```python
from build123d import *

# Parameters (mm, degrees)
SKETCH_1_W              = 306
SKETCH_1_H              = 175
EXTRUDE_1_DEPTH         = 2
SKETCH_2_R              = 110
SKETCH_2_W              = 10
SKETCH_2_H              = 80
CUT_EXTRUDE_1_DEPTH     = 177.264715698
FILLET_1_R              = 5
HOLE_WIZARD_3_2_3_2_1_D = 3.2
HOLE_WIZARD_3_2_3_2_2_D = 3.2
CUT_EXTRUDE_2_DEPTH     = 10
FILLET_2_R              = 2
FILLET_2_OF_MIRROR_3_R  = 2


with BuildPart() as part:
    # 草图1 → 凸台-拉伸1 (new body)
    with BuildSketch(Plane.XY):
        Rectangle(SKETCH_1_W, SKETCH_1_H)
    extrude(amount=EXTRUDE_1_DEPTH)

    # 草图2 → 切除-拉伸1 (cut, through all)
    with BuildSketch(Plane.XY.offset(2)):
        with Locations((0, 87.5)):
            Circle(SKETCH_2_R)
        with Locations((-148, -7.5)):
            Rectangle(SKETCH_2_W, SKETCH_2_H)
        with Locations((148, -7.5)):
            Rectangle(SKETCH_2_W, SKETCH_2_H)
    extrude(amount=-CUT_EXTRUDE_1_DEPTH, mode=Mode.SUBTRACT)

    # 圆角1
    fillet_1_edges = [part.edges().sort_by_distance(p)[0] for p in [
        (143, -47.5, 1),
        (143, 32.5, 1),
        (-143, 32.5, 1),
        (-143, -47.5, 1),
    ]]
    fillet(fillet_1_edges, radius=FILLET_1_R)

    # Ø3.2 (3.2) 直径孔1 (through all)
    with Locations(Plane(origin=(-147, 82.5, 2), x_dir=(1, 0, 0), z_dir=(0, 0, 1))):
        with Locations((0, 0), (0, -20)):
            hole_wizard_3_2_3_2_1 = Hole(HOLE_WIZARD_3_2_3_2_1_D / 2)

    # 镜向1: Ø3.2 (3.2) 直径孔1 across plane
    add(hole_wizard_3_2_3_2_1.mirror(Plane(origin=(0, 0, 0), x_dir=(0, 0, 1), z_dir=(1, 0, 0))), mode=Mode.SUBTRACT)

    # Ø3.2 (3.2) 直径孔2 (through all)
    with Locations(Plane(origin=(-113, -81.5, 2), x_dir=(1, 0, 0), z_dir=(0, 0, 1))):
        with Locations((0, 0), (20, 0)):
            hole_wizard_3_2_3_2_2 = Hole(HOLE_WIZARD_3_2_3_2_2_D / 2)

    # 镜向2: Ø3.2 (3.2) 直径孔2 across plane
    add(hole_wizard_3_2_3_2_2.mirror(Plane(origin=(0, 0, 0), x_dir=(0, 0, 1), z_dir=(1, 0, 0))), mode=Mode.SUBTRACT)

    # 草图7 → 切除-拉伸2 (cut)
    with BuildSketch(Plane.XY.offset(2)):
        with BuildLine():
            Line((-138, 77.5), (-138, 37.5))
            Line((-138, 37.5), (-116.553428589, 58.946571411))
            ThreePointArc((-116.553428589, 58.946571411), (-118.431897329, 68.163875903), (-119.582607431, 77.5))
            Line((-119.582607431, 77.5), (-138, 77.5))
        make_face()
        with BuildLine():
            Line((-127.46644704, 33.891417336), (-113.324311416, 48.03355296))
            ThreePointArc((-113.324311416, 48.03355296), (-107.177013369, 33.526971501), (-99.182175793, 19.950788272))
            Line((-99.182175793, 19.950788272), (-99.182175793, 5.607146089))
            Line((-99.182175793, 5.607146089), (-127.46644704, 33.891417336))
        make_face()
        Polygon((-133, 25.282834672), (-99.182175793, -8.534989535), (-99.182175793, -58.302319282), align=None)
        Polygon((-133, 3.952734845), (-133, -53.571693723), (-113, -45.479868176), align=None)
        Polygon((-133, -64.359159143), (-133, -72.5), (-104.225383435, -72.5), (-111.10343515, -55.5), align=None)
        with BuildLine():
            Line((-89.182175793, 7.209654871), (-89.182175793, -48.302319282))
            Line((-89.182175793, -48.302319282), (-67.900763938, -11.441832693))
            ThreePointArc((-67.900763938, -11.441832693), (-79.093185457, -2.74559831), (-89.182175793, 7.209654871))
        make_face()
        Polygon((-91.605707885, -72.5), (-80.058702502, -52.5), (-31.605707885, -72.5), align=None)
        Polygon((-75.014735912, -43.763593595), (-65.014735912, -26.44308552), (-5.396488671, -72.5), align=None)
        Polygon((-5.396488671, -59.863531439), (-5.396488671, -29.863531439), (-48.657493674, -26.44308552), align=None)
    cut_extrude_2 = extrude(amount=-CUT_EXTRUDE_2_DEPTH, mode=Mode.SUBTRACT)

    # 圆角2
    fillet_2_edges = [part.edges().sort_by_distance(p)[0] for p in [
        (-89.182175793, 7.209654871, 1),
        (-67.900763938, -11.441832693, 1),
        (-89.182175793, -48.302319282, 1),
        (-31.605707885, -72.5, 1),
        (-91.605707885, -72.5, 1),
        (-80.058702502, -52.5, 1),
        (-48.657493674, -26.44308552, 1),
        (-5.396488671, -29.863531439, 1),
        (-5.396488671, -59.863531439, 1),
        (-5.396488671, -72.5, 1),
        (-75.014735912, -43.763593595, 1),
        (-65.014735912, -26.44308552, 1),
        (-104.225383435, -72.5, 1),
        (-133, -72.5, 1),
        (-133, -64.359159143, 1),
        (-111.10343515, -55.5, 1),
        (-99.182175793, 5.607146089, 1),
        (-127.46644704, 33.891417336, 1),
        (-113.324311416, 48.03355296, 1),
        (-99.182175793, 19.950788272, 1),
        (-133, 3.952734845, 1),
        (-113, -45.479868176, 1),
        (-133, -53.571693723, 1),
        (-99.182175793, -58.302319282, 1),
        (-133, 25.282834672, 1),
        (-99.182175793, -8.534989535, 1),
        (-138, 77.5, 1),
        (-119.582607431, 77.5, 1),
        (-116.553428589, 58.946571411, 1),
        (-138, 37.5, 1),
    ]]
    fillet(fillet_2_edges, radius=FILLET_2_R)

    # 镜向3: 切除-拉伸2 across plane
    add(cut_extrude_2.mirror(Plane(origin=(0, 0, 0), x_dir=(0, 0, 1), z_dir=(1, 0, 0))), mode=Mode.SUBTRACT)

    # 圆角2 of 镜向3
    fillet_2_of_mirror_3_edges = [part.edges().sort_by_distance(p)[0] for p in [
        (89.182175793, 7.209654871, 1),
        (67.900763938, -11.441832693, 1),
        (89.182175793, -48.302319282, 1),
        (31.605707885, -72.5, 1),
        (91.605707885, -72.5, 1),
        (80.058702502, -52.5, 1),
        (48.657493674, -26.44308552, 1),
        (5.396488671, -29.863531439, 1),
        (5.396488671, -59.863531439, 1),
        (5.396488671, -72.5, 1),
        (75.014735912, -43.763593595, 1),
        (65.014735912, -26.44308552, 1),
        (104.225383435, -72.5, 1),
        (133, -72.5, 1),
        (133, -64.359159143, 1),
        (111.10343515, -55.5, 1),
        (99.182175793, 5.607146089, 1),
        (127.46644704, 33.891417336, 1),
        (113.324311416, 48.03355296, 1),
        (99.182175793, 19.950788272, 1),
        (133, 3.952734845, 1),
        (113, -45.479868176, 1),
        (133, -53.571693723, 1),
        (99.182175793, -58.302319282, 1),
        (133, 25.282834672, 1),
        (99.182175793, -8.534989535, 1),
        (138, 77.5, 1),
        (119.582607431, 77.5, 1),
        (116.553428589, 58.946571411, 1),
        (138, 37.5, 1),
    ]]
    fillet(fillet_2_of_mirror_3_edges, radius=FILLET_2_OF_MIRROR_3_R)


solid = part.part
```
Here's how the part is built. I have some questions about the finished solid (model axes, mm). Coordinates: 2 decimals unless noted, no trailing zeros. Loops run counter-clockwise (first coordinate to the right, second up) from the corner with the lowest first, then second, coordinate; pieces in that order, holes last. Notation, with made-up numbers: (45.5, -40) - (104.5, -40) arc R14 ccw to (104.5, -25) - close; hole circle Ø5 at (42.5, 72.5). An arc over 180 degrees is marked (long way). Answer as CSV lines item,"result".
Q1. If we section it at B-B, the plane x = 0: Write out the boundary of the cut face in (y, z), and give its area (3 significant figures).
Response:
outline,"(-87.5, 0) - (-22.5, 0) - (-22.5, 2) - (-87.5, 2) - close"
area,"130 mm2"
Q2. If I drill on L1, parallel to X at y = -81.5, z = 1.05; L2, parallel to Y at x = 101.5, z = 1.15; L3, parallel to X at y = 76, z = 1.45, over which ranges is the centre line in solid material (lowest first)? Write a range as [from, to].
Response:
L1,"[-153, -114.6], [-111.4, -94.6], [-91.4, 91.4], [94.6, 111.4], [114.6, 153]"
L2,"[-87.5, -50], [-6.22, 8.46], [23.49, 45.1]"
L3,"[-153, -137.94], [-119.47, -109.4], [109.4, 119.47], [137.94, 153]"
Q3. We'd pull the mould along X, two halves only. Please class faces 1 (the face through (115.99, -16.76, 1.01)), 2 (the face through (-2, -38, 0)): pulls with the +X half, pulls with the -X half, needs draft (parallel to the pull), parting line crosses it, or undercut.
Response:
face 1,"undercut"
face 2,"needs draft"
Q4. If we section it at A-A, the plane z = 1.3: Give the number of separate pieces and of enclosed holes in the cut face, and give its area (3 significant figures).
Response:
separate pieces,"1"
enclosed holes,"26"
area,"22,400 mm2"
